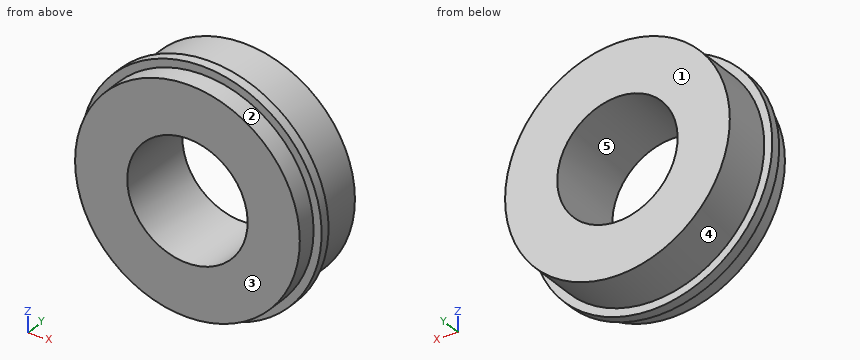
from build123d import *

# Parameters (mm, degrees)
F0_W = 5
F0_H = 4


with BuildPart() as f1:
    # F0 (on Right) → F1 (revolve)
    with BuildSketch(Plane.YZ):
        Polygon((-10, 56), (-20, 56), (-20, 30), (20, 30), (20, 56), (-5, 56), align=None)
        with Locations((-7.5, 58)):
            Rectangle(F0_W, F0_H)
    revolve(axis=Axis((0, -1.266651, 0), (0, -1, 0)))


solid = f1.part
Can you work these out from the model? Positions are in its coordinate system, mm. Face numbers are marked on the shaded views. A direction names the side the tool comes from. Coordinates: 2 decimals unless noted, no trailing zeros. Write each loop counter-clockwise with the first axis right and the second up, starting at its lowest first coordinate (ties: lowest second). Pieces come first, ordered by that corner, then holes. Notation, with made-up numbers: (7, 66.5) -> (15, 66.5) arc R20 cw to (15, 83.5) -> close; hole circle Ø9 at (43, 78.25). An arc over 180 degrees is marked (long way). Answer as CSV lines item,"result".
1) If we section it at A-A on x = 0: Please give me the cut outline in (y, z).
Check result:
outline,"(-20, -56) -> (-10, -56) -> (-10, -60) -> (-5, -60) -> (-5, -56) -> (20, -56) -> (20, -30) -> (-20, -30) -> close; (-20, 30) -> (20, 30) -> (20, 56) -> (-5, 56) -> (-5, 60) -> (-10, 60) -> (-10, 56) -> (-20, 56) -> close"
2) If we section it at B-B on z = 0: Please give me the cut outline in (x, y).
Check result:
outline,"(-60, -10) -> (-56, -10) -> (-56, -20) -> (-30, -20) -> (-30, 20) -> (-56, 20) -> (-56, -5) -> (-60, -5) -> close; (30, -20) -> (56, -20) -> (56, -10) -> (60, -10) -> (60, -5) -> (56, -5) -> (56, 20) -> (30, 20) -> close"
3) If we section it at C-C on y = 10: Please give me the cut outline in (x, z).
Check result:
outline,"circle Ø112 at (0, 0); hole circle Ø60 at (0, 0)"
4) On a 3-axis mill with a long thin cutter (end or side, diameter ignored), from which of +Z, -Z, +X, -X, +Y, -Y can I reach the whole of each face in a straight line? I mean the marked faces 1 and 2. Say none if no direction works.
Check result:
face 1,"+Z, -Z, +X, -X, +Y"
face 2,"-Y"
5) If we mould it in two halves opening along Z, with no side actions, what happens to the marked faces 3, 4 and 5? For each: +Z half, -Z half, draft (parallel to the pull), parting line (faces both ways), or undercut.
Check result:
face 3,"draft"
face 4,"parting line"
face 5,"undercut"
6) Will these pins go through, and if not, where does the flat tip stop? P1, Ø12, axis at y = -11.5, z = -0.5, coming from the +X side; P2, Ø1.5, axis at x = 20.5, z = 20.5, coming from the +Y side; P3, Ø4, axis at x = 42.5, y = -7, coming from the -Z side; P4, Ø8, axis at x = -42, z = -47, coming from the -Y side.
Check result:
P1,"x = 60"
P2,"through"
P3,"z = -44.27"
P4,"y = -10"
7) If I drill on line 1 (X direction, y = 10, z = 0); line 2 (Z direction, x = 0, y = -9), over which ranges is the centre line in solid material (lowest first)? Write a range as from..to.
Check result:
line 1,"-56..-30, 30..56"
line 2,"-60..-30, 30..60"
8) If we section it at D-D on x = 40: Please give me the cut outline in (y, z).
Check result:
outline,"(-20, -39.19) -> (-10, -39.19) -> (-10, -44.72) -> (-5, -44.72) -> (-5, -39.19) -> (20, -39.19) -> (20, 39.19) -> (-5, 39.19) -> (-5, 44.72) -> (-10, 44.72) -> (-10, 39.19) -> (-20, 39.19) -> close"
